from build123d import *

# Parameters (mm, degrees)
BOSS_EXTRUDE1_DEPTH = 127
SKETCH2_R           = 14.2748
CUT_EXTRUDE1_DEPTH  = 4.175


with BuildPart() as part:
    # Sketch1 → Boss-Extrude1 (new body, symmetric)
    with BuildSketch(Plane(origin=(0, 0, 0), x_dir=(1, 0, 0), z_dir=(0, 1, 0))):
        Polygon((0, 0), (3.175, 0), (3.175, 347.6625), (176.2125, 347.6625), (176.2125, 350.8375), (0, 350.8375), align=None)
    extrude(amount=BOSS_EXTRUDE1_DEPTH, both=True)

    # Sketch2 → Cut-Extrude1 (cut, through all)
    with BuildSketch(Plane(origin=(3.175, 0, 0), x_dir=(0, 0, -1), z_dir=(1, 0, 0))):
        with Locations((309.5625, -88.9)):
            Circle(SKETCH2_R)
        with Locations((309.5625, 88.9)):
            Circle(SKETCH2_R)
        with Locations((38.1, -88.9)):
            Circle(SKETCH2_R)
        with Locations((38.1, 88.9)):
            Circle(SKETCH2_R)
    extrude(amount=-CUT_EXTRUDE1_DEPTH, mode=Mode.SUBTRACT)


solid = part.part
Here's how the part is built. I have some questions about the finished solid (model axes, mm). A direction names the side the tool comes from. Give positions to 0.01 mm unless a question says otherwise; leave off trailing zeros. Order: outer loops, then holes, each group sorted by start corner. A loop starts at its lowest first (then second) coordinate and runs counter-clockwise, first axis right, second up. Notation, with made-up numbers: (-7.5, 60) -> (43.5, 60) arc R18 ccw to (43.5, 94) -> close; hole circle Ø9 at (-14, -1.5). An arc over 180 degrees is marked (long way). One line per item, written item: value. Start each with the question number.
1. I need wall thicknesses on probe 1 along Z at (x, y) = (1, -88); probe 2 along Y at (x, z) = (1.35, -38.1); probe 3 along X at (y, z) = (-77.5, -333) (3 decimals). Which ranges of each line are inside material? Lowest first, please. Write a range as from..to.
2. Imagine slicing it at B-B, the plane z = -38.1. List the corners of the cut face in (x, y) for me (3 decimals), plus the area to 3 significant figures.
3. Will these pins go through, and if not, where does the flat tip stop? pin 1 Ø23 at (y, z) = (-88.9, -309.56) entering from +X; pin 2 Ø1 at (y, z) = (65.5, -58.5) entering from +X (3 decimals).
4. Imagine slicing it at D-D, the plane x = 104.5. List the corners of the cut face in (y, z) for me, plus the area to 3 significant figures.
5. We'd pull the mould along Y, two halves only. Please class faces 1 (the face through (1.6, -88.3, -295.3)), 2 (the face through (0, 2, -178)), 3 (the face through (3, -127, -176)): released by +Y, released by -Y, zero draft, split by the parting line, or undercut.
6. Imagine slicing it at C-C, the plane y = 28. List the corners of the cut face in (x, z) for me (1 decimal).
7. For faces 4 (the face through (1.6, 89.5, -295.3)), 5 (the face through (3.175, 2, -171)), which set-ups out of +Z, -Z, +X, -X, +Y, -Y let a thin tool reach every point of the face, with its end or its side?
8. Imagine slicing it at A-A, the plane y = -88.9. List the corners of the cut face in (x, z) for me (1 decimal).
Values follow:
1. probe 1: z = -350.84..-323.81, -295.32..-52.35, -23.85..0
1. probe 2: y = -127..-103.17, -74.63..74.63, 103.17..127
1. probe 3: x = 0..3.175
2. outline: (0, -127) -> (3.175, -127) -> (3.175, -103.175) -> (0, -103.175) -> close; (0, -74.625) -> (3.175, -74.625) -> (3.175, 74.625) -> (0, 74.625) -> close; (0, 103.175) -> (3.175, 103.175) -> (3.175, 127) -> (0, 127) -> close
2. area: 625 mm2
3. pin 1: passes through
3. pin 2: stops at x = 3.175
4. outline: (-127, -350.84) -> (127, -350.84) -> (127, -347.66) -> (-127, -347.66) -> close
4. area: 806 mm2
5. face 1: undercut
5. face 2: zero draft
5. face 3: released by -Y
6. outline: (0, -350.8) -> (176.2, -350.8) -> (176.2, -347.7) -> (3.2, -347.7) -> (3.2, 0) -> (0, 0) -> close
7. face 4: +X, -X
7. face 5: +Z, +X, +Y, -Y
8. outline: (0, -350.8) -> (176.2, -350.8) -> (176.2, -347.7) -> (3.2, -347.7) -> (3.2, -323.8) -> (0, -323.8) -> close; (0, -295.3) -> (3.2, -295.3) -> (3.2, -52.4) -> (0, -52.4) -> close; (0, -23.8) -> (3.2, -23.8) -> (3.2, 0) -> (0, 0) -> close
